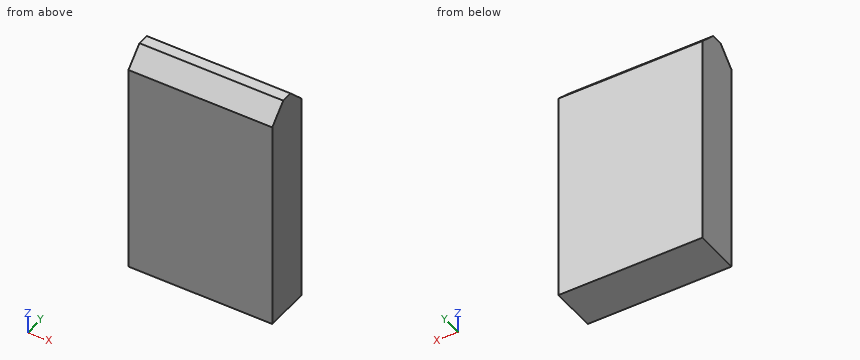
from build123d import *

# Parameters (mm, degrees)
SKETCH_1_W      = 25
SKETCH_1_H      = 40
EXTRUDE_1_DEPTH = 8
CHAMFER_1_SIZE  = 3


with BuildPart() as part:
    # 草图1 → 凸台-拉伸1 (new body)
    with BuildSketch(Plane(origin=(0, 0, 0), x_dir=(1, 0, 0), z_dir=(0, 1, 0))):
        with Locations((12.5, 20)):
            Rectangle(SKETCH_1_W, SKETCH_1_H)
    extrude(amount=EXTRUDE_1_DEPTH)

    # 倒角1
    chamfer_1_edges = [part.edges().sort_by_distance(p)[0] for p in [
        (12.5, 0, 0),
        (12.5, 8, 0),
    ]]
    chamfer(chamfer_1_edges, length=CHAMFER_1_SIZE)


solid = part.part
Model file for the job. Use its own axes, mm. Give positions to 0.01 mm unless a question says otherwise; leave off trailing zeros. Loops run counter-clockwise (first coordinate to the right, second up) from the corner with the lowest first, then second, coordinate; pieces in that order, holes last. Notation, with made-up numbers: (-11.75, 36.5) - (27.25, 36.5) arc R25 ccw to (27.25, 62.5) - close; hole circle Ø10 at (-33, -17). An arc over 180 degrees is marked (long way). Use one line per item in the form item = value.
(1) Cut at A-A (x = 4.5). Give the cut face in (y, z), then the cut area to 3 significant figures.
Determined:
outline = (0, -40) - (8, -40) - (8, -3) - (5, 0) - (3, 0) - (0, -3) - close
area = 311 mm^2
(2) Cut at B-B (y = 7.25). Give the cut face in (x, z), then the cut area to 3 significant figures.
Determined:
outline = (0, -40) - (25, -40) - (25, -2.25) - (0, -2.25) - close
area = 944 mm^2
(3) Cut at C-C (y = 0.5). Give the cut face in (x, z).
Determined:
outline = (0, -40) - (25, -40) - (25, -2.5) - (0, -2.5) - close
(4) Drill centre lines: L1, parallel to Z at x = 16, y = 2.25; L2, parallel to Z at x = 19, y = 5.5. Where is each one in solid material? Low to high.
Determined:
L1 = -40 to -0.75
L2 = -40 to -0.5
